Could you check a few things on this model? Use its own coordinates, in mm. A direction names the side the tool comes from. Coordinates: 2 decimals unless noted, no trailing zeros. Order: outer loops, then holes, each group sorted by start corner. A loop starts at its lowest first (then second) coordinate and runs counter-clockwise, first axis right, second up. Notation, with made-up numbers: (3.25, 26) -> (26.25, 26) arc R20 cw to (26.25, 61) -> close; hole circle Ø4 at (67, -37.75). An arc over 180 degrees is marked (long way). Put each result on its own line as item: value. Start each with the question number.
Q1. If we section it at C-C (y = 3): Please give me the cut outline in (x, z).
Q2. If we section it at A-A (z = 0): Please give me the cut outline in (x, y), and give its area (3 significant figures).
Q3. Please list where these lines run through material, in increasing order: line 1 along Y through (x, z) = (1, 1.8); line 2 along Y through (x, z) = (-1, -0.65); line 3 along Z through (x, y) = (0.1, 8).
Q4. Will this pin go through, and if not, where does the flat tip stop? pin 1 (2 mm diameter, centred on x = -0.5, z = 1.5, fed in from +Y).
Q5. If we section it at D-D (x = -1.2): Please give me the cut outline in (y, z).
Q6. If we section it at B-B (x = 0): Please give me the cut outline in (y, z), and give its area (3 significant figures).
Q7. For faces 1 (the face through (0.54, 9.94, 2.44)), 2 (the face through (0, 6, 2)), 3 (the face through (0, 17, 1)), which set-ups out of +Z, -Z, +X, -X, +Y, -Y let a thin tool reach every point of the face, with its end or its side?
Solid Edge part; units mm, degrees
sketch "Sketch1" plane through (0, 0, 0) normal (0, -1, 0) x (1, 0, 0)
  circle A0 centre (0, 0) radius 1.5
extrude "Protrusion1" add sketch "Sketch1" against normal blind 6
sketch "Sketch2" plane through (0, 6, 0) normal (0, 1, 0) x (-1, 0, 0)
  circle A0 centre (0, 0) radius 2.5
extrude "ExtrudedProtrusion_2" add sketch "Sketch2" along normal blind 8
sketch "Sketch3" plane through (0, 14, 0) normal (0, 1, 0) x (-1, 0, 0)
  circle A0 centre (0, 0) radius 1
extrude "ExtrudedProtrusion_3" add sketch "Sketch3" along normal blind 7
The answers:
1. outline: circle Ø3 at (0, 0)
2. outline: (-2.5, 6) -> (-1.5, 6) -> (-1.5, 0) -> (1.5, 0) -> (1.5, 6) -> (2.5, 6) -> (2.5, 14) -> (1, 14) -> (1, 21) -> (-1, 21) -> (-1, 14) -> (-2.5, 14) -> close
2. area: 72.0 mm^2
3. line 1: 6 to 14
3. line 2: 0 to 14
3. line 3: -2.5 to 2.5
4. pin 1: y = 21
5. outline: (0, -0.9) -> (6, -0.9) -> (6, -2.19) -> (14, -2.19) -> (14, 2.19) -> (6, 2.19) -> (6, 0.9) -> (0, 0.9) -> close
6. outline: (0, -1.5) -> (6, -1.5) -> (6, -2.5) -> (14, -2.5) -> (14, -1) -> (21, -1) -> (21, 1) -> (14, 1) -> (14, 2.5) -> (6, 2.5) -> (6, 1.5) -> (0, 1.5) -> close
6. area: 72.0 mm^2
7. face 1: +Y, -Y
7. face 2: -Y
7. face 3: +Y
